Build history of the part. All positions in model axes, mm. Give positions to 0.01 mm unless a question says otherwise; leave off trailing zeros. Write each loop counter-clockwise with the first axis right and the second up, starting at its lowest first coordinate (ties: lowest second). Pieces come first, ordered by that corner, then holes. Notation, with made-up numbers: (29, -36) -> (60, -36) arc R15 ccw to (60, -15) -> close; hole circle Ø2 at (18.5, 75). An arc over 180 degrees is marked (long way). Put each result on its own line as item: value. Start each with the question number.
Item 1: Two-plate mould, pull along X, no slides. Class faces 1 (the cylindrical face through (29.33, 0.482, 51.617)), 2 (the cylindrical face through (21.802, 1.014, -6.277)), 3 (the cylindrical face through (34.4, 1.01, -54.43)), 4 (the flat face through (-35, 1, 1)): pulls with the +X half, pulls with the -X half, needs draft (parallel to the pull), parting line crosses it, or undercut.
Item 2: Slice it at C-C, the plane x = 18.5. List the corners of the cut face in (y, z).
Item 3: Slice it at A-A, the plane z = 50. List the corners of the cut face in (x, y).
Item 4: Flat gauge pins, fed straight in: pin 1 Ø7 at (x, z) = (-20, -12) entering from -Y (3 decimals); pin 2 Ø12 at (x, z) = (-0.5, -37) entering from -Y; pin 3 Ø4.5 at (x, z) = (-30, 50) entering from +Y. Where does each tip first touch, or does it go through?
Item 5: Drill centre lines: line 1 along X through (y, z) = (0.5, -50); line 2 along X through (y, z) = (0.5, -12); line 3 along Z through (x, y) = (31, 1.15). Where is each one in solid material? Low to high.
Item 6: Slice it at B-B, the plane z = 31. List the corners of the cut face in (x, y).
Item 7: Slice it at D-D, the plane y = 1.65. Give the number of separate pieces and of enclosed holes in the cut face, plus the area to 3 significant figures.
```python
from build123d import *

# Parameters (mm, degrees)
FACE_PLATE_W           = 70
FACE_PLATE_H           = 110
FACE_PLATE_EXT_DEPTH   = 2
BUTTONS_R              = 6
BUTTONS_R_2            = 3.55
BUTTONS_CUT_DEPTH      = 10
M3_TOP_SCREW_R         = 1.75
M3_TOP_SCREW_CUT_DEPTH = 10
FILLET1_R              = 2
FILLET2_R              = 2
FILLET3_R              = 2
FILLET4_R              = 2


with BuildPart() as part:
    # Face Plate → Face Plate Ext (new body)
    with BuildSketch(Plane(origin=(0, 0, 0), x_dir=(1, 0, 0), z_dir=(0, 1, 0))):
        Rectangle(FACE_PLATE_W, FACE_PLATE_H)
    extrude(amount=FACE_PLATE_EXT_DEPTH)

    # Buttons → Buttons CUT (cut)
    with BuildSketch(Plane(origin=(0, 2, 0), x_dir=(1, 0, 0), z_dir=(0, 1, 0))):
        with Locations(Location((-20, 12, 0), (0, 0, 270))):
            Circle(BUTTONS_R)
        with Locations(Location((20, 12, 0), (0, 0, 270))):
            Circle(BUTTONS_R)
        with Locations(Location((-20, -18, 0), (0, 0, 270))):
            Circle(BUTTONS_R_2)
        with Locations(Location((-20, -44, 0), (0, 0, 270))):
            Circle(BUTTONS_R_2)
        with Locations(Location((-20, 40, 0), (0, 0, 270))):
            Circle(BUTTONS_R_2)
        with Locations(Location((20, -18, 0), (0, 0, 270))):
            Circle(BUTTONS_R_2)
        with Locations(Location((20, -44, 0), (0, 0, 270))):
            Circle(BUTTONS_R_2)
        with Locations(Location((20, 40, 0), (0, 0, 270))):
            Circle(BUTTONS_R)
        with Locations(Location((0, -31, 0), (0, 0, 270))):
            Circle(BUTTONS_R)
        with Locations(Location((0, -3.5, 0), (0, 0, 270))):
            Circle(BUTTONS_R)
    extrude(amount=-BUTTONS_CUT_DEPTH, mode=Mode.SUBTRACT)

    # M3 Top Screw → M3 Top Screw CUT (cut)
    with BuildSketch(Plane(origin=(0, 2, 0), x_dir=(1, 0, 0), z_dir=(0, 1, 0))):
        with Locations(Location((-30, 50, 0), (0, 0, 270))):
            Circle(M3_TOP_SCREW_R)
        with Locations(Location((30, 50, 0), (0, 0, 270))):
            Circle(M3_TOP_SCREW_R)
        with Locations(Location((-30, -50, 0), (0, 0, 270))):
            Circle(M3_TOP_SCREW_R)
        with Locations(Location((30, -50, 0), (0, 0, 270))):
            Circle(M3_TOP_SCREW_R)
    extrude(amount=-M3_TOP_SCREW_CUT_DEPTH, mode=Mode.SUBTRACT)

    # M3 Head Top CUT cone 1 section (through the dimple's axis) → M3 Head Top CUT (revolve, cut)
    with BuildSketch(Plane(origin=(-30, 2, -50), x_dir=(0, 0, 1), z_dir=(1, 0, 0))):
        Polygon((0, 0), (2.8, 0), (0, 2.8), align=None)
    revolve(axis=Axis((-30, 2, -50), (0, -1, 0)), mode=Mode.SUBTRACT)

    # M3 Head Top CUT cone 2 section (through the dimple's axis) → M3 Head Top CUT cone 2 (revolve, cut)
    with BuildSketch(Plane(origin=(30, 2, -50), x_dir=(0, 0, 1), z_dir=(1, 0, 0))):
        Polygon((0, 0), (2.8, 0), (0, 2.8), align=None)
    revolve(axis=Axis((30, 2, -50), (0, -1, 0)), mode=Mode.SUBTRACT)

    # M3 Head Top CUT cone 3 section (through the dimple's axis) → M3 Head Top CUT cone 3 (revolve, cut)
    with BuildSketch(Plane(origin=(30, 2, 50), x_dir=(0, 0, 1), z_dir=(1, 0, 0))):
        Polygon((0, 0), (2.8, 0), (0, 2.8), align=None)
    revolve(axis=Axis((30, 2, 50), (0, -1, 0)), mode=Mode.SUBTRACT)

    # M3 Head Top CUT cone 4 section (through the dimple's axis) → M3 Head Top CUT cone 4 (revolve, cut)
    with BuildSketch(Plane(origin=(-30, 2, 50), x_dir=(0, 0, 1), z_dir=(1, 0, 0))):
        Polygon((0, 0), (2.8, 0), (0, 2.8), align=None)
    revolve(axis=Axis((-30, 2, 50), (0, -1, 0)), mode=Mode.SUBTRACT)

    # Fillet1
    fillet1_edges = [part.edges().sort_by_distance(p)[0] for p in [
        (-35, 1, -55),
    ]]
    fillet(fillet1_edges, radius=FILLET1_R)

    # Fillet2
    fillet2_edges = [part.edges().sort_by_distance(p)[0] for p in [
        (35, 1, -55),
    ]]
    fillet(fillet2_edges, radius=FILLET2_R)

    # Fillet3
    fillet3_edges = [part.edges().sort_by_distance(p)[0] for p in [
        (35, 1, 55),
    ]]
    fillet(fillet3_edges, radius=FILLET3_R)

    # Fillet4
    fillet4_edges = [part.edges().sort_by_distance(p)[0] for p in [
        (-35, 1, 55),
    ]]
    fillet(fillet4_edges, radius=FILLET4_R)


solid = part.part
```
Values follow:
1. face 1: undercut
1. face 2: undercut
1. face 3: pulls with the +X half
1. face 4: pulls with the -X half
2. outline: (0, -55) -> (2, -55) -> (2, -45.81) -> (0, -45.81) -> close; (0, -34.19) -> (2, -34.19) -> (2, -17.81) -> (0, -17.81) -> close; (0, -6.19) -> (2, -6.19) -> (2, 14.78) -> (0, 14.78) -> close; (0, 21.22) -> (2, 21.22) -> (2, 40.78) -> (0, 40.78) -> close; (0, 47.22) -> (2, 47.22) -> (2, 55) -> (0, 55) -> close
3. outline: (-35, 0) -> (-31.75, 0) -> (-31.75, 0.95) -> (-32.8, 2) -> (-35, 2) -> close; (-28.25, 0) -> (28.25, 0) -> (28.25, 0.95) -> (27.2, 2) -> (-27.2, 2) -> (-28.25, 0.95) -> close; (31.75, 0) -> (35, 0) -> (35, 2) -> (32.8, 2) -> (31.75, 0.95) -> close
4. pin 1: through
4. pin 2: y = 0
4. pin 3: y = 1.45
5. line 1: -35 to -31.75, -28.25 to 28.25, 31.75 to 35
5. line 2: -35 to -26, -14 to 14, 26 to 35
5. line 3: -55 to -51.67, -48.33 to 48.33, 51.67 to 55
6. outline: (-35, 0) -> (-6, 0) -> (-6, 2) -> (-35, 2) -> close; (6, 0) -> (35, 0) -> (35, 2) -> (6, 2) -> close
7. separate pieces: 1
7. enclosed holes: 14
7. area: 6,860 mm2
